from build123d import *

# Parameters (mm, degrees)
F1_DEPTH    = 130
F2_T1_DEPTH = 154.4948974279
F3_T1_DEPTH = 154.4948974279
F4_R        = 5


# Not quite as in the source:
# - a fillet or chamfer that OpenCascade refuses, or shapes differently, is made with other operations: its cross-section is extruded or revolved along the edge and cut away or added


with BuildPart() as f1:
    # F0 (on Right) → F1 (new body)
    with BuildSketch(Plane.YZ):
        Polygon((1.0352761804, 3.8637033052), (0, 0), (120, 0), (120, 4), (5.2129014914, 4), (44.0560821698, 148.9647238196), (40.1923788647, 150), align=None)
        Polygon((-30, 0), (0, 0), (1.0352761804, 3.8637033052), (-30, 12.1795804946), (-30, 4.0079755444), align=None)
    extrude(amount=F1_DEPTH)

    # F2: fillet of radius 5 on 1 edges, made by hand

    # F2_s2 → F2_t1 (cut)
    with BuildSketch(Plane.YZ.offset(-12.2474487139)):
        with BuildLine():
            ThreePointArc((44.0560821698, 148.9647238196), (40.8315018491, 148.0307814801), (38.9244296722, 145.2679491924))
            Line((38.9244296722, 145.2679491924), (40.1923788647, 150))
            Line((40.1923788647, 150), (44.0560821698, 148.9647238196))
        make_face()
    extrude(amount=F2_T1_DEPTH, mode=Mode.SUBTRACT)

    # F3: fillet of radius 5 on 1 edges, made by hand

    # F3_s2 → F3_t1 (cut)
    with BuildSketch(Plane.YZ.offset(-12.2474487139)):
        with BuildLine():
            ThreePointArc((115.1010205144, 4), (118.2632981746, 2.8729833462), (120, 0))
            Line((120, 0), (120, 4))
            Line((120, 4), (115.1010205144, 4))
        make_face()
    extrude(amount=F3_T1_DEPTH, mode=Mode.SUBTRACT)

    # F4
    f4_edges = [f1.edges().sort_by_distance(p)[0] for p in [
        (65, -30, 12.17958),
    ]]
    fillet(f4_edges, radius=F4_R)


solid = f1.part
Can you work these out from the model? Positions are in its coordinate system, mm. A direction names the side the tool comes from. Round coordinates to 2 decimals unless told otherwise and drop trailing zeros. Order: outer loops, then holes, each group sorted by start corner. A loop starts at its lowest first (then second) coordinate and runs counter-clockwise, first axis right, second up. Notation, with made-up numbers: (40, 20.5) - (44, 20.5) arc R22 cw to (44, 40.5) - close; hole circle Ø9 at (-30, -37.75). An arc over 180 degrees is marked (long way). Answer in a Markdown table with one row per item.
(1) For P1, Ø4, axis at x = 61.5, y = -13, coming from the -Z side; P2, Ø1, axis at x = 89.5, z = 102.5, coming from the +Y side; P3, Ø6, axis at x = 110, z = 44.5, coming from the +Y side; P4, Ø12, axis at x = 92.5, z = 47, coming from the +Y side, each with a flat end and sliding along its axis, tell me the tip position at first contact or that it passes through.
From the geometry:
| item | result |
|---|---|
| P1 | stops at z = 0 |
| P2 | stops at y = 31.74 |
| P3 | stops at y = 16.87 |
| P4 | stops at y = 18.34 |
(2) Which directions (+Z, -Z, +X, -X, +Y, -Y) give clear straight access to the entire face, cutting with the end or side of a thin tool? Please do faces 4 (the face through (64.09, 24.363, 75.468)), 5 (the face through (64, -30, 3)).
From the geometry:
| item | result |
|---|---|
| face 4 | +X, -X, +Y |
| face 5 | +Z, -Z, +X, -X, -Y |
(3) Suppose I cut it at A-A, the plane y = 22. Please give me the cut outline in (x, z), plus the area to 3 significant figures.
From the geometry:
| item | result |
|---|---|
| outline | (0, 0) - (130, 0) - (130, 4) - (0, 4) - close; (0, 66.65) - (130, 66.65) - (130, 82.11) - (0, 82.11) - close |
| area | 2,530 mm2 |
(4) Suppose I cut it at C-C, the plane y = 95.5. Please give me the cut outline in (x, z), plus the area to 3 significant figures.
From the geometry:
| item | result |
|---|---|
| outline | (0, 0) - (130, 0) - (130, 4) - (0, 4) - close |
| area | 520 mm2 |
(5) Suppose I cut it at B-B, the plane x = 112. Please give me the cut outline in (y, z), plus the area to 3 significant figures.
From the geometry:
| item | result |
|---|---|
| outline | (-30, 0) - (120, 0) arc R5 ccw to (115.1, 4) - (5.21, 4) - (44.06, 148.96) arc R5 ccw to (38.92, 145.27) - (1.04, 3.86) - (-23.71, 10.49) arc R5 ccw to (-30, 5.66) - close |
| area | 1,310 mm2 |
(6) Suppose I cut it at D-D, the plane z = 123. Please give me the cut outline in (x, y), plus the area to 3 significant figures.
From the geometry:
| item | result |
|---|---|
| outline | (0, 32.96) - (130, 32.96) - (130, 37.1) - (0, 37.1) - close |
| area | 538 mm2 |
(7) Please list where these lines run through material, in increasing order: L1, parallel to Z at x = 84.5, y = 84; L2, parallel to Y at x = 23, z = 76.5; L3, parallel to Z at x = 121, y = -17.5. Write a range as from..to.
From the geometry:
| item | result |
|---|---|
| L1 | z = 0..4 |
| L2 | y = 20.5..24.64 |
| L3 | z = 0..8.83 |
(8) If we mould it in two halves opening along Y, with no side actions, what happens to faces 1 (the face through (64, 61, 4)), 2 (the face through (64.09, -11.16, 7.13)), 3 (the face through (64.09, 118.23, 2.9))? For each: released by +Y, released by -Y, zero draft, split by the parting line, or undercut.
From the geometry:
| item | result |
|---|---|
| face 1 | zero draft |
| face 2 | undercut |
| face 3 | released by +Y |
